from build123d import *

# Parameters (mm, degrees)
F0_R     = 11
F1_DEPTH = 7


with BuildPart() as f1:
    # F0 (on Top) → F1 (new body)
    with BuildSketch(Plane.XY):
        with BuildLine():
            ThreePointArc((9.994443, 30.333333), (9.998611, 30.16669), (10, 30))
            ThreePointArc((10, 30), (-0.16669, 20.001389), (-9.994443, 30.333333))
            Line((-9.994443, 30.333333), (-10.709236, 8.901461))
            ThreePointArc((-10.709236, 8.901461), (-11.37633, 6.568127), (-13.063509, 4.82374))
            Line((-13.063509, 4.82374), (-31.266659, -6.511225))
            ThreePointArc((-31.266659, -6.511225), (-21.125814, -6.257604), (-15.980762, -15))
            ThreePointArc((-15.980762, -15), (-17.405056, -20.143663), (-21.272216, -23.822108))
            Line((-21.272216, -23.822108), (-2.354273, -13.725201))
            ThreePointArc((-2.354273, -13.725201), (0, -13.136255), (2.354273, -13.725201))
            Line((2.354273, -13.725201), (21.272216, -23.822108))
            ThreePointArc((21.272216, -23.822108), (17.320508, -10), (31.266659, -6.511225))
            Line((31.266659, -6.511225), (28.860169, -5.012722))
            Line((28.860169, -5.012722), (13.063509, 4.82374))
            ThreePointArc((13.063509, 4.82374), (11.37633, 6.568127), (10.709236, 8.901461))
            Line((10.709236, 8.901461), (10.17232, 25))
            Line((10.17232, 25), (9.994443, 30.333333))
        make_face()
        Circle(F0_R, mode=Mode.SUBTRACT)
        with BuildLine():
            ThreePointArc((-9.994443, 30.333333), (-0.16669, 20.001389), (10, 30))
            ThreePointArc((10, 30), (9.998611, 30.16669), (9.994443, 30.333333))
            ThreePointArc((9.994443, 30.333333), (9.614774, 32.748841), (8.660254, 35))
            ThreePointArc((8.660254, 35), (-2.426821, 39.701059), (-9.994443, 30.333333))
        make_face()
        with BuildLine():
            ThreePointArc((-15.980762, -15), (-21.125814, -6.257604), (-31.266659, -6.511225))
            ThreePointArc((-31.266659, -6.511225), (-34.641016, -20), (-21.272216, -23.822108))
            ThreePointArc((-21.272216, -23.822108), (-17.405056, -20.143663), (-15.980762, -15))
        make_face()
        with BuildLine():
            ThreePointArc((32.987055, -7.864745), (32.164004, -7.140769), (31.266659, -6.511225))
            ThreePointArc((31.266659, -6.511225), (17.320508, -10), (21.272216, -23.822108))
            ThreePointArc((21.272216, -23.822108), (31.124425, -23.575706), (35.980762, -15))
            ThreePointArc((35.980762, -15), (35.202013, -11.131081), (32.987055, -7.864745))
        make_face()
        with BuildLine():
            ThreePointArc((8.660254, 35), (9.614774, 32.748841), (9.994443, 30.333333))
            Line((9.994443, 30.333333), (10.17232, 25))
            Line((10.17232, 25), (17.468503, 18.338699))
            Line((17.468503, 18.338699), (13.411126, 16.494436))
            Line((13.411126, 16.494436), (27.48383, 3.646278))
            Line((27.48383, 3.646278), (23.627748, 2.462574))
            Line((23.627748, 2.462574), (28.860169, -5.012722))
            Line((28.860169, -5.012722), (31.266659, -6.511225))
            ThreePointArc((31.266659, -6.511225), (32.164004, -7.140769), (32.987055, -7.864745))
            Line((32.987055, -7.864745), (28.558979, 0.540369))
            Line((28.558979, 0.540369), (33.061294, 2.263841))
            Line((33.061294, 2.263841), (20.695962, 15.572305))
            Line((20.695962, 15.572305), (25.122192, 17.693207))
            Line((25.122192, 17.693207), (8.660254, 35))
        make_face()
    extrude(amount=F1_DEPTH)


solid = f1.part
Check sheet for the modelled part. Datum: model origin and axes. Units: mm. A direction names the side the tool comes from. Give positions to 0.01 mm unless a question says otherwise; leave off trailing zeros. Write each loop counter-clockwise with the first axis right and the second up, starting at its lowest first coordinate (ties: lowest second). Pieces come first, ordered by that corner, then holes. Notation, with made-up numbers: (-24, 69.25) -> (21, 69.25) arc R5 ccw to (21, 74.25) -> close; hole circle Ø11 at (-0.5, 22). An arc over 180 degrees is marked (long way). Use one line per item in the form item = value. Start each with the question number.
1. Section check D-D (x = -29.5). Record the cut outline in (y, z).
2. Section check A-A (x = 0). Record the cut outline in (y, z), and give its area (3 significant figures).
3. Thickness scan on line 1 along Y through (x, z) = (0, 3.25); line 2 along Y through (x, z) = (21.5, 4.75); line 3 along X through (y, z) = (13, 4.25). Record the ranges inside material, lowest first. Write a range as from..to.
4. Section check C-C (z = 3.5). Record the cut outline in (x, y).
5. Mould release check, pull along Y, two halves, no side actions. Record for faces 5 (the flat face through (26.207, -1.223, 3.451)), 6 (the cylindrical face through (-34.75, -19.81, 3.45)), 7 (the cylindrical face through (-0.034, -13.136, 3.451)): pulls with the +Y half, pulls with the -Y half, needs draft (parallel to the pull), parting line crosses it, or undercut.
6. Go/stop test with flat-tipped pins: P1, Ø3, axis at y = 20, z = 6, coming from the -X side; P2, Ø1.5, axis at x = -23.5, z = 4.5, coming from the +Y side; P3, Ø2, axis at y = -11, z = 3.5, coming from the -X side. Record where each tip stops, or that it passes through.
7. Section check B-B (y = -4). Record the cut outline in (x, z), and give its area (3 significant figures).
8. Access from +Z, -Z, +X, -X, +Y, -Y to the whole of each face (thin tool, end or side, straight path). Record for faces 1 (the flat face through (-11.946, -18.844, 3.451)), 2 (the flat face through (-22.038, -0.764, 3.451)), 3 (the flat face through (30.8, 1.4, 3.5)), 4 (the flat face through (25.58, 3.06, 3.45)).
Conclusion:
q1.outline = (-24.36, 0) -> (-5.41, 0) -> (-5.41, 7) -> (-24.36, 7) -> close
q2.outline = (-13.14, 0) -> (-11, 0) -> (-11, 7) -> (-13.14, 7) -> close; (11, 0) -> (40, 0) -> (40, 7) -> (11, 7) -> close
q2.area = 218 mm²
q3.line_1 = -13.14..-11, 11..40
q3.line_2 = -23.94..-0.43, 9.11..14.71, 15.96..21.5
q3.line_3 = -10.57..10.57, 17.24..23.09
q4.outline = (-31.27, -6.51) arc R10 ccw to (-21.27, -23.82) -> (-2.35, -13.73) arc R5 cw to (2.35, -13.73) -> (21.27, -23.82) arc R10 ccw to (35.98, -15) arc R10 ccw to (32.99, -7.86) -> (28.56, 0.54) -> (33.06, 2.26) -> (20.7, 15.57) -> (25.12, 17.69) -> (8.66, 35) arc R10 ccw to (-9.99, 30.33) -> (-10.71, 8.9) arc R5 cw to (-13.06, 4.82) -> close; hole circle Ø22 at (0, 0); hole (10.17, 25) -> (10.71, 8.9) arc R5 ccw to (13.06, 4.82) -> (28.86, -5.01) -> (23.63, 2.46) -> (27.48, 3.65) -> (13.41, 16.49) -> (17.47, 18.34) -> close
q5.face_5 = undercut
q5.face_6 = parting line crosses it
q5.face_7 = pulls with the -Y half
q6.P1 = -10.39
q6.P2 = -1.21
q6.P3 = -35.52
q7.outline = (-27.23, 0) -> (-10.25, 0) -> (-10.25, 7) -> (-27.23, 7) -> close; (10.25, 0) -> (27.23, 0) -> (27.23, 7) -> (10.25, 7) -> close; (28.15, 0) -> (30.95, 0) -> (30.95, 7) -> (28.15, 7) -> close
q7.area = 257 mm²
q8.face_1 = +Z, -Z, -Y
q8.face_2 = +Z, -Z, -X, +Y
q8.face_3 = +Z, -Z, +X
q8.face_4 = +Z, -Z
